from build123d import *

# Parameters (mm, degrees)
F0_R     = 50
F0_R_2   = 46
F0_R_3   = 43.6
F0_R_4   = 5
F1_DEPTH = 2
F2_DEPTH = 30
F0_R_5   = 2.2
F3_DEPTH = 20
F4_SIZE  = 4


with BuildPart() as f1:
    # F0 (on Top) → F1 (new body)
    with BuildSketch(Plane.XY):
        Circle(F0_R)
        Circle(F0_R_2, mode=Mode.SUBTRACT)
        Circle(F0_R_2)
        Circle(F0_R_3, mode=Mode.SUBTRACT)
        Circle(F0_R_3)
        Circle(F0_R_4, mode=Mode.SUBTRACT)
    extrude(amount=F1_DEPTH)

    # F0 (on Top) → F2 (join)
    with BuildSketch(Plane.XY):
        Circle(F0_R_2)
        Circle(F0_R_3, mode=Mode.SUBTRACT)
    extrude(amount=F2_DEPTH)

    # F0 (on Top) → F3 (join)
    with BuildSketch(Plane.XY):
        Circle(F0_R_4)
        Circle(F0_R_5, mode=Mode.SUBTRACT)
    extrude(amount=F3_DEPTH)

    # F4
    f4_edges = [f1.edges().sort_by_distance(p)[0] for p in [
        (-5, 0, 2),
        (-43.6, 0, 2),
    ]]
    chamfer(f4_edges, length=F4_SIZE)


solid = f1.part
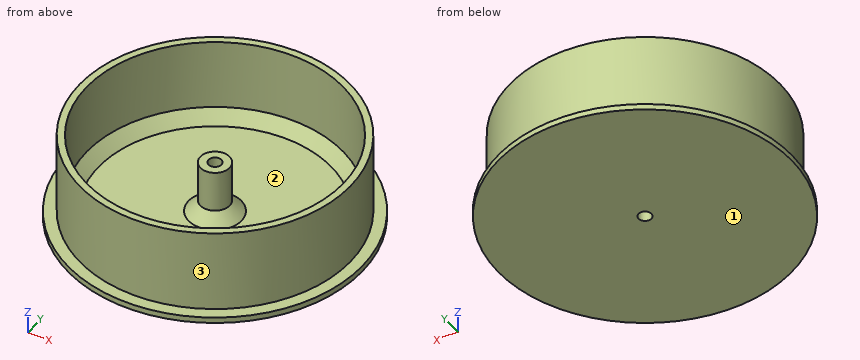
Could you check a few things on this model? Use its own coordinates, in mm. Face numbers are marked on the shaded views. Give positions to 0.01 mm unless a question says otherwise; leave off trailing zeros. Order: outer loops, then holes, each group sorted by start corner. A loop starts at its lowest first (then second) coordinate and runs counter-clockwise, first axis right, second up.
1. I need wall thicknesses on L1, parallel to Y at x = 0, z = 13.25; L2, parallel to X at y = 0, z = 23; L3, parallel to Z at x = 7.5, y = -34.5. Which ranges of each line are inside material? Lowest first, please.
2. Suppose I cut it at C-C (z = 18). List the corners of the cut face in (x, y) for me.
3. Suppose I cut it at A-A (y = 0). List the corners of the cut face in (x, z) for me, plus the area to 3 significant figures.
4. Suppose I cut it at D-D (z = 23.5). List the corners of the cut face in (x, y) for me.
5. We'd pull the mould along X, two halves only. Please class the marked faces 1, 2 and 3: pulls with the +X half, pulls with the -X half, needs draft (parallel to the pull), parting line crosses it, or undercut.
6. Will these pins go through, and if not, where does the flat tip stop? P1, Ø4, axis at x = 0, y = 0, coming from the +Z side; P2, Ø1, axis at x = 20.5, z = 16, coming from the -Y side; P3, Ø4, axis at y = 34, z = 21, coming from the -X side; P4, Ø12, axis at x = -24, z = 13, coming from the +Y side.
Solved:
1. L1: y = -46 to -43.6, -5 to -2.2, 2.2 to 5, 43.6 to 46
1. L2: x = -46 to -43.6, 43.6 to 46
1. L3: z = 0 to 2
2. outline: circle Ø92 at (0, 0); circle Ø10 at (0, 0); hole circle Ø87.2 at (0, 0); hole circle Ø4.4 at (0, 0)
3. outline: (-50, 0) - (-2.2, 0) - (-2.2, 20) - (-5, 20) - (-5, 6) - (-9, 2) - (-39.6, 2) - (-43.6, 6) - (-43.6, 30) - (-46, 30) - (-46, 2) - (-50, 2) - close; (2.2, 0) - (50, 0) - (50, 2) - (46, 2) - (46, 30) - (43.6, 30) - (43.6, 6) - (39.6, 2) - (9, 2) - (5, 6) - (5, 20) - (2.2, 20) - close
3. area: 458 mm2
4. outline: circle Ø92 at (0, 0); hole circle Ø87.2 at (0, 0)
5. face 1: needs draft
5. face 2: undercut
5. face 3: parting line crosses it
6. P1: passes through
6. P2: stops at y = -41.42
6. P3: stops at x = -33.05
6. P4: stops at y = 42.33
